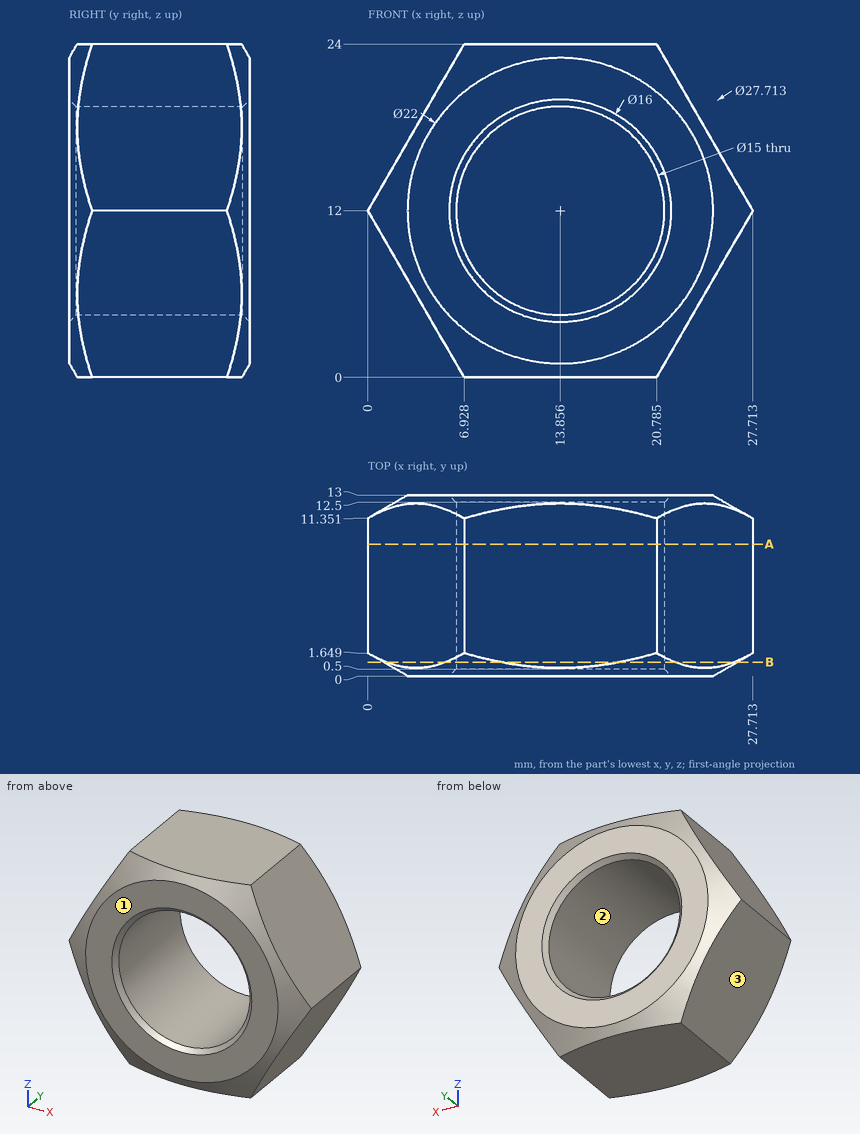
Could you check a few things on this drawing? It's one solid part, dimensions in mm from its lowest x, y, z. Coordinates: 2 decimals unless noted, no trailing zeros. Order: outer loops, then holes, each group sorted by start corner. A loop starts at its lowest first (then second) coordinate and runs counter-clockwise, first axis right, second up.
1) We'd pull the mould along Z, two halves only. Please class the marked faces 1, 2 and 3: +Z half, -Z half, draft (parallel to the pull), parting line (faces both ways), or undercut.
2) Will these pins go through, and if not, where does the flat tip stop? pin 1 (4 mm diameter, centred on y = 6, z = 4.5, fed in from -X) (1 decimal); pin 2 (5 mm diameter, centred on y = 7, z = 3, fed in from +X); pin 3 (3 mm diameter, centred on y = 3, z = 16.5, fed in from +X).
3) Imagine slicing it at A-A on y = 9.5. List the corners of the cut face in (x, z) for me (1 decimal), and give its area (3 significant figures).
4) I need wall thicknesses on line 1 (Z direction, x = 12.5, y = 1.5); line 2 (X direction, y = 2, z = 6.25) (1 decimal); line 3 (Z direction, x = 12, y = 9.5). Which ranges of each line are inside material? Lowest first, please.
5) Imagine slicing it at B-B on y = 1. List the corners of the cut face in (x, z) for me (1 decimal).
Response values:
1. face 1: draft
1. face 2: undercut
1. face 3: -Z half
2. pin 1: stops at x = 3.2
2. pin 2: stops at x = 23.96
2. pin 3: stops at x = 25.98
3. outline: (0, 12) - (6.9, 0) - (20.8, 0) - (27.7, 12) - (20.8, 24) - (6.9, 24) - close; hole circle Ø15 at (13.9, 12)
3. area: 322 mm2
4. line 1: z = 0 to 4.62, 19.38 to 24
4. line 2: x = 3.3 to 9, 18.7 to 24.4
4. line 3: z = 0 to 4.73, 19.27 to 24
5. outline: (1.3, 9.7) - (5.6, 2.3) arc R12.7 ccw to (9.6, 0) - (18.1, 0) arc R12.7 ccw to (22.1, 2.3) - (26.4, 9.7) arc R12.7 ccw to (26.4, 14.3) - (22.1, 21.7) arc R12.7 ccw to (18.1, 24) - (9.6, 24) arc R12.7 ccw to (5.6, 21.7) - (1.3, 14.3) arc R12.7 ccw to start; hole circle Ø15 at (13.9, 12)
